Source: three-view drawing plus pictorial views. Frame: mm from the lowest corner of the part. A direction names the side the tool comes from. Give positions to 0.01 mm unless a question says otherwise; leave off trailing zeros. Loops run counter-clockwise (first coordinate to the right, second up) from the corner with the lowest first, then second, coordinate; pieces in that order, holes last. Notation, with made-up numbers: (-27.75, -10) - (28.25, -10) arc R27 ccw to (28.25, 12) - close; hole circle Ø11 at (52.5, 39.25). An arc over 180 degrees is marked (long way). Put each result on its own line as item: value.
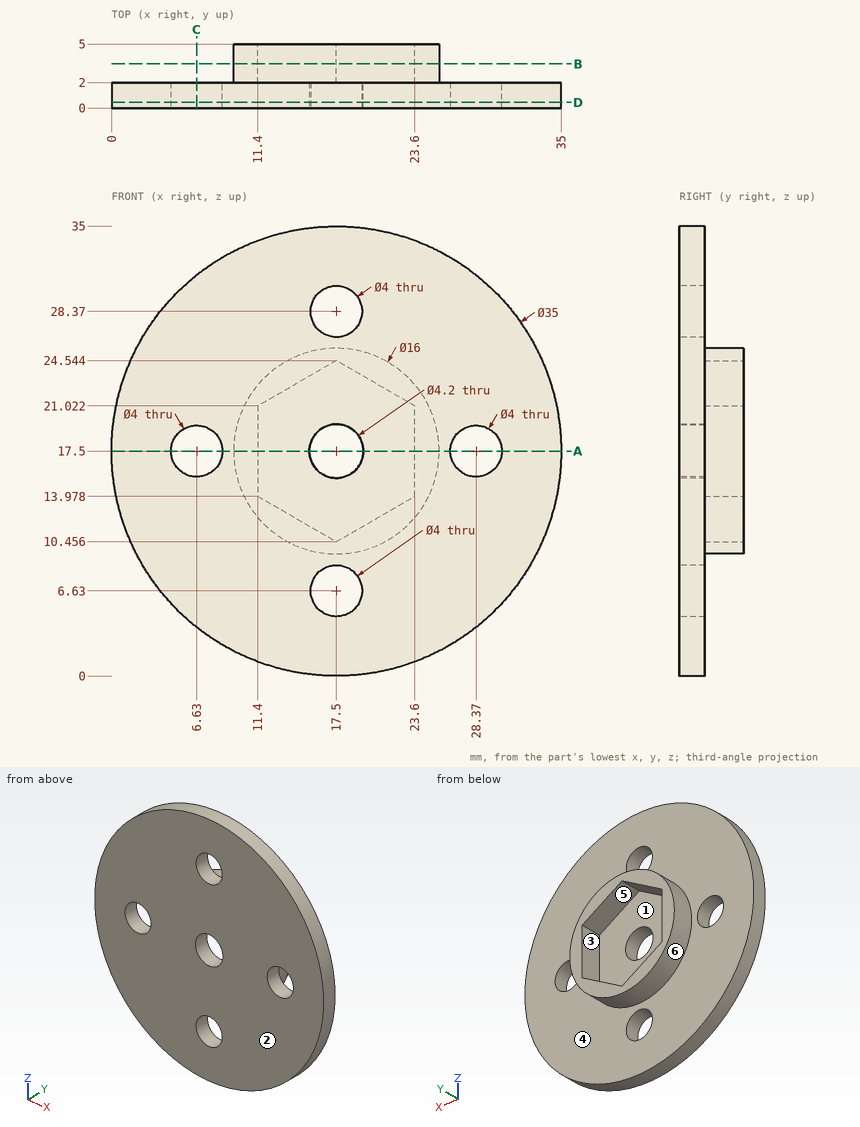
1) Section query D-D, the plane y = 0.45. Output: boundary loops of the cut face in (x, z), plus the area to 3 significant figures.
Check result:
outline: circle Ø35 at (17.5, 17.5); hole circle Ø4 at (6.63, 17.5); hole circle Ø4.2 at (17.5, 17.5); hole circle Ø4 at (17.5, 6.63); hole circle Ø4 at (17.5, 28.37); hole circle Ø4 at (28.37, 17.5)
area: 898 mm²
2) Section query B-B, the plane y = 3.45. Output: boundary loops of the cut face in (x, z).
Check result:
outline: circle Ø16 at (17.5, 17.5); hole (11.4, 13.98) - (17.5, 10.46) - (23.6, 13.98) - (23.6, 21.02) - (17.5, 24.54) - (11.4, 21.02) - close
3) Section query A-A, the plane z = 17.5. Output: boundary loops of the cut face in (x, y).
Check result:
outline: (0, 0) - (4.63, 0) - (4.63, 2) - (0, 2) - close; (8.63, 0) - (15.4, 0) - (15.4, 2) - (11.4, 2) - (11.4, 5) - (9.5, 5) - (9.5, 2) - (8.63, 2) - close; (19.6, 0) - (26.37, 0) - (26.37, 2) - (25.5, 2) - (25.5, 5) - (23.6, 5) - (23.6, 2) - (19.6, 2) - close; (30.37, 0) - (35, 0) - (35, 2) - (30.37, 2) - close
4) Mould query, pull axis Z, two halves, no side actions, for the marked faces 3, 4, 5 and 6. Classes: pulls with the +Z half, pulls with the -Z half, needs draft (parallel to the pull), parting line crosses it, or undercut.
Check result:
face 3: undercut
face 4: needs draft
face 5: undercut
face 6: parting line crosses it
5) Section query C-C, the plane x = 6.63. Output: boundary loops of the cut face in (y, z) (1 decimal).
Check result:
outline: (0, 3.8) - (2, 3.8) - (2, 15.5) - (0, 15.5) - close; (0, 19.5) - (2, 19.5) - (2, 31.2) - (0, 31.2) - close
6) Pin query (flat end, axial travel): P1, Ø1.5, axis at y = 3.5, z = 16.5, coming from the +X side; P2, Ø10, axis at x = 20.5, z = 20, coming from the +Y side; P3, Ø3.5, axis at x = 17.5, z = 6.63, coming from the -Y side; P4, Ø1.5, axis at y = 4, z = 16.5, coming from the -X side. Return the tip coordinate at first contact, or that it passes through.
Check result:
P1: x = 25.5
P2: y = 5
P3: through
P4: x = 9.5
7) Material intervals for line 1 along X through (y, z) = (0.9, 17.5); line 2 along Z through (x, y) = (16, 1.2) (1 decimal), sorted ascending. Write a range as [from, to].
Check result:
line 1: [0, 4.63], [8.63, 15.4], [19.6, 26.37], [30.37, 35]
line 2: [0.1, 5.3], [8, 16], [19, 27], [29.7, 34.9]
8) Access query for the marked faces 1 and 2. Directions: +Z, -Z, +X, -X, +Y, -Y. A direction counts if a zero-diameter tool reaches every point of the face in a straight line with its end or side. Return the directions, or none.
Check result:
face 1: +Y
face 2: +Z, -Z, +X, -X, -Y
